from build123d import *

# Parameters (mm, degrees)
SKETCH1_W                 = 25.4
SKETCH1_H                 = 12.7
BOSS_EXTRUDE1_DEPTH       = 12.7
SKETCH2_R                 = 3.571875
SKETCH3_R                 = 0.3175
CUT_EXTRUDE2_REACH        = 23.997
F_2_56_TAPPED_HOLE2_D     = 2.1844
F_2_56_TAPPED_HOLE2_DEPTH = 3.302
F_2_56_TAPPED_HOLE2_TIP   = 0.656259968
CIRPATTERN1_COUNT         = 3


with BuildPart() as part:
    # Sketch1 → Boss-Extrude1 (new body)
    with BuildSketch(Plane(origin=(0, 0, 0), x_dir=(1, 0, 0), z_dir=(0, 1, 0))):
        Rectangle(SKETCH1_W, SKETCH1_H)
    extrude(amount=BOSS_EXTRUDE1_DEPTH)

    # Sketch2 → Cut-Loft2 section 0
    with BuildSketch(Plane(origin=(12.7, 0, 0), x_dir=(0, 0, -1), z_dir=(1, 0, 0))):
        with Locations((0, 6.35)):
            Circle(SKETCH2_R)
    # Sketch3 → Cut-Loft2 section 1
    with BuildSketch(Plane.ZY.offset(12.7)):
        with Locations((0, 6.35)):
            Circle(SKETCH3_R)
    loft(mode=Mode.SUBTRACT)

    # Cut-Extrude2: up to this face of the body (flat: up to its plane)
    cut_extrude2_end = Plane(part.part.faces().sort_by_distance((0, 6.35, -6.35))[0])
    # Sketch6 → Cut-Extrude2 (cut, up to the picked face)
    with BuildSketch(Plane.XY.offset(6.35), mode=Mode.PRIVATE) as cut_extrude2_sk1:
        Polygon((-11.938, 12.7), (11.938, 12.7), (11.938, 9.798636115), (-11.938, 6.739523615), align=None)
    cut_extrude2_tool1 = split(extrude(cut_extrude2_sk1.sketch, amount=-CUT_EXTRUDE2_REACH, mode=Mode.PRIVATE), bisect_by=cut_extrude2_end, keep=Keep.BOTH, mode=Mode.PRIVATE)
    add(cut_extrude2_tool1.solids().sort_by(Axis((-1.373668, 10.396539, 6.35), (0, 0, -1)))[0], mode=Mode.SUBTRACT)

    # #2-56 Tapped Hole2
    with Locations(Plane(origin=(-1.042364388, 8.135526928, 0), x_dir=(0.9918916863822601, 0.12708612231772706, 0), z_dir=(-0.12708612231772703, 0.99189168638226, 0))):
        with Locations((1.050885295, 3.385522314)):
            Hole(F_2_56_TAPPED_HOLE2_D / 2, depth=F_2_56_TAPPED_HOLE2_DEPTH)
            with Locations((0, 0, -(F_2_56_TAPPED_HOLE2_DEPTH + F_2_56_TAPPED_HOLE2_TIP / 2))):  # 118° drill point
                Cone(0, F_2_56_TAPPED_HOLE2_D / 2, F_2_56_TAPPED_HOLE2_TIP, mode=Mode.SUBTRACT)

    # Sketch26 → #2-56 Tapped Hole3 (revolve, cut)
    with BuildSketch(Plane(origin=(-12.7, 2.54, 0), x_dir=(0, 0, 1), z_dir=(0, 1, 0))):
        Polygon((0, 0), (0, 3.958259968), (1.0922, 3.302), (1.0922, 0), align=None)
    f_2_56_tapped_hole3 = revolve(axis=Axis((-19.05, 2.54, 0), (1, 0, 0)), mode=Mode.SUBTRACT)

    # CirPattern1: #2-56 Tapped Hole3 ×3 about axis
    cirpattern1_axis = Axis((0, 6.35, 0), (1, 0, 0))
    for i in range(1, CIRPATTERN1_COUNT):
        add(f_2_56_tapped_hole3.rotate(cirpattern1_axis, i * 360 / CIRPATTERN1_COUNT), mode=Mode.SUBTRACT)


solid = part.part
Design review of the part built by this model. Coordinates are the model's own, in mm. A direction names the side the tool comes from. Give positions to 0.01 mm unless a question says otherwise; leave off trailing zeros. Loops run counter-clockwise (first coordinate to the right, second up) from the corner with the lowest first, then second, coordinate; pieces in that order, holes last. Notation, with made-up numbers: M -13,8.5 L 16,8.5 A11 ccw 16,23.5 Z; hole C 64,1.25 d4. An arc over 180 degrees is marked long. One line per question, with ' | ' between items. Start each with the question number.
1. Add section B-B (z = 4.75). Write out the cut boundary in (x, y), plus the area to 3 significant figures.
2. Add section A-A (y = 11.5). Write out the cut boundary in (x, z).
3. Insertion check: P1, Ø1.3, axis at y = 2.54, z = 0, coming from the -X side. The pin has a flat end and moves straight along its axis. Give the tip position at first contact, or say it passes through.
4. To check wall thickness, follow L1, parallel to Z at x = -11.3, y = 2.54; L2, parallel to X at y = 11, z = 0.25; L3, parallel to Z at x = 6.75, y = 7.5. State the ranges of each line that lie inside material, in increasing order.
5. Add section C-C (y = 6.35). Give the number of separate pieces and of enclosed holes in the cut face, plus the area to 3 significant figures.
6. For faces 4 (the face through (-12.32, 9.32, -3.54)), 5 (the face through (0.45, 4.45, -3.2)), 6 (the face through (11.938, 11, 0)), 7 (the face through (-12.7, 6, 2)), list the 3-axis set-ups (+Z, -Z, +X, -X, +Y, -Y) from which the entire face can be reached by the end or side of a thin tool; tool diameter is ignored.
7. The part is to be moulded in two halves that separate along Z. For faces 1 (the face through (-0.178, 4.474, 0.417)), 2 (the face through (0.17, 8.29, 3.29)), 3 (the face through (0, 3, -6.35)), say which applies: released by +Z, released by -Z, zero draft, split by the parting line, or undercut.
8. Add section D-D (x = 8.5). Write out the cut boundary in (y, z).
Worked out:
1) outline: M -12.7,0 L 12.7,0 L 12.7,12.7 L 11.94,12.7 L 11.94,9.8 L -11.94,6.74 L -11.94,12.7 L -12.7,12.7 Z | area: 217 mm²
2) outline: M -12.7,-6.35 L -11.94,-6.35 L -11.94,6.35 L -12.7,6.35 Z; M 11.94,-6.35 L 12.7,-6.35 L 12.7,6.35 L 11.94,6.35 Z
3) P1: stops at x = -9.13
4) L1: z = -6.35 to -1.09, 1.09 to 6.35 | L2: x = -12.7 to -11.94, 11.94 to 12.7 | L3: z = -6.35 to -2.56, 2.56 to 6.35
5) separate pieces: 2 | enclosed holes: 1 | area: 220 mm²
6) face 4: -X | face 5: none | face 6: +Z, -Z, +Y | face 7: +Z, -Z, -X, +Y, -Y
7) face 1: undercut | face 2: zero draft | face 3: released by -Z
8) outline: M 0,-6.35 L 9.36,-6.35 L 9.36,-0.39 A3.03 cw long 9.36,0.39 L 9.36,6.35 L 0,6.35 Z
